The model under review builds one solid part; all positions refer to its coordinate system, in mm. Round coordinates to 2 decimals unless told otherwise and drop trailing zeros. Loops run counter-clockwise (first coordinate to the right, second up) from the corner with the lowest first, then second, coordinate; pieces in that order, holes last. Notation, with made-up numbers: M 24.25,22.25 L 48.25,22.25 A28 cw 48.25,45.25 Z; hole C 66.5,8 d5. An arc over 180 degrees is marked long. Return JSON: item names as keys, results as strings. Group by question number.
Q1. Draft analysis for pull direction Y (two halves, no side actions). For faces 1 (the face through (-103, 406.4, 13)), 2 (the face through (-100.447, 74.932, 16.008)), 3 (the face through (-103, 206, 25.4)), state which applies: pulls with the +Y half, pulls with the -Y half, needs draft (parallel to the pull), parting line crosses it, or undercut.
Q2. Consider section C-C (x = -171.45). State the section outline as (y, z) points.
Q3. To check wall thickness, follow line 1 along X through (y, z) = (387.35, 5) (3 decimals); line 2 along X through (y, z) = (275.5, 15.5); line 3 along Z through (x, y) = (-26.5, 111.5). State the ranges of each line that lie inside material, in increasing order.
Q4. Consider section B-B (y = 261). State the section outline as (x, z) points.
Q5. Clearance check with flat-ended pins moving along their axes: pin 1 Ø10 at (x, y) = (-146, 136) entering from -Z; pin 2 Ø17 at (x, y) = (-114.5, 239) entering from +Z. State where each tip first meets the part, or that it passes through.
Q6. Consider section A-A (z = 14). Count the separate pieces of the cut face and the enclosed holes in it, and give its area (3 significant figures).
Q7. Consider section D-D (y = 217.5). State the section outline as (x, z) points.
from build123d import *

# Parameters (mm, degrees)
F0_W     = 203.2
F0_H     = 406.4
F1_DEPTH = 25.4
F3_DEPTH = 19.05
F4_R     = 3.175
F5_DEPTH = 25.401


with BuildPart() as f1:
    # F0 (on Top) → F1 (new body)
    with BuildSketch(Plane.XY):
        with Locations((-101.6, 203.2)):
            Rectangle(F0_W, F0_H)
    extrude(amount=F1_DEPTH)

    # F2 (on face) → F3 (cut)
    with BuildSketch(Plane.XY.offset(25.4)):
        with BuildLine():
            ThreePointArc((-162.33913, 21.369951), (-101.6, 36.836287), (-40.86087, 21.369951))
            ThreePointArc((-40.86087, 21.369951), (-15.019951, 28.98913), (-22.63913, 54.830049))
            ThreePointArc((-22.63913, 54.830049), (-101.6, 74.936287), (-180.56087, 54.830049))
            ThreePointArc((-180.56087, 54.830049), (-188.180049, 28.98913), (-162.33913, 21.369951))
        make_face()
        with BuildLine():
            ThreePointArc((-162.233016, 84.869862), (-101.493885, 100.336199), (-40.754755, 84.869862))
            ThreePointArc((-40.754755, 84.869862), (-14.913836, 92.489042), (-22.533016, 118.329961))
            ThreePointArc((-22.533016, 118.329961), (-101.493885, 138.436199), (-180.454755, 118.329961))
            ThreePointArc((-180.454755, 118.329961), (-188.073935, 92.489042), (-162.233016, 84.869862))
        make_face()
        with BuildLine():
            ThreePointArc((-162.126901, 148.369773), (-101.387771, 163.83611), (-40.64864, 148.369773))
            ThreePointArc((-40.64864, 148.369773), (-14.807721, 155.988953), (-22.426901, 181.829872))
            ThreePointArc((-22.426901, 181.829872), (-101.387771, 201.93611), (-180.34864, 181.829872))
            ThreePointArc((-180.34864, 181.829872), (-187.96782, 155.988953), (-162.126901, 148.369773))
        make_face()
        with BuildLine():
            ThreePointArc((-162.020787, 211.869685), (-101.281656, 227.336021), (-40.542526, 211.869685))
            ThreePointArc((-40.542526, 211.869685), (-14.701607, 219.488864), (-22.320787, 245.329783))
            ThreePointArc((-22.320787, 245.329783), (-101.281656, 265.436021), (-180.242526, 245.329783))
            ThreePointArc((-180.242526, 245.329783), (-187.861706, 219.488864), (-162.020787, 211.869685))
        make_face()
        with BuildLine():
            ThreePointArc((-161.914672, 275.369596), (-101.175541, 290.835933), (-40.436411, 275.369596))
            ThreePointArc((-40.436411, 275.369596), (-14.595492, 282.988776), (-22.214672, 308.829695))
            ThreePointArc((-22.214672, 308.829695), (-101.175541, 328.935933), (-180.136411, 308.829695))
            ThreePointArc((-180.136411, 308.829695), (-187.755591, 282.988776), (-161.914672, 275.369596))
        make_face()
        with BuildLine():
            ThreePointArc((-161.808557, 338.869507), (-101.069427, 354.335844), (-40.330296, 338.869507))
            ThreePointArc((-40.330296, 338.869507), (-14.489377, 346.488687), (-22.108557, 372.329606))
            ThreePointArc((-22.108557, 372.329606), (-101.069427, 392.435844), (-180.030296, 372.329606))
            ThreePointArc((-180.030296, 372.329606), (-187.649476, 346.488687), (-161.808557, 338.869507))
        make_face()
    extrude(amount=-F3_DEPTH, mode=Mode.SUBTRACT)

    # F4 (on face) → F5 (cut, through all)
    with BuildSketch(Plane.XY.offset(25.4)):
        with Locations((-184.15, 387.35)):
            Circle(F4_R)
        with Locations((-19.05, 387.35)):
            Circle(F4_R)
        with Locations((-184.15, 12.7)):
            Circle(F4_R)
        with Locations((-19.05, 12.7)):
            Circle(F4_R)
    extrude(amount=-F5_DEPTH, mode=Mode.SUBTRACT)


solid = f1.part
Values:
{
 "1": {"face 1": "pulls with the +Y half", "face 2": "undercut", "face 3": "needs draft"},
 "2": {"outline": "M 0,0 L 406.4,0 L 406.4,25.4 L 376.68,25.4 L 376.68,6.35 L 336.56,6.35 L 336.56,25.4 L 313.23,25.4 L 313.23,6.35 L 273.05,6.35 L 273.05,25.4 L 249.78,25.4 L 249.78,6.35 L 209.55,6.35 L 209.55,25.4 L 186.33,25.4 L 186.33,6.35 L 146.05,6.35 L 146.05,25.4 L 122.88,25.4 L 122.88,6.35 L 82.55,6.35 L 82.55,25.4 L 59.43,25.4 L 59.43,6.35 L 19.05,6.35 L 19.05,25.4 L 0,25.4 Z"},
 "3": {"line 1": "x = -203.2 to -187.325, -180.975 to -22.225, -15.875 to 0", "line 2": "x = -203.2 to -180.37, -161.67 to -40.68, -21.98 to 0", "line 3": "z = 0 to 6.35"},
 "4": {"outline": "M -203.2,0 L 0,0 L 0,25.4 L -63.27,25.4 L -63.27,6.35 L -139.3,6.35 L -139.3,25.4 L -203.2,25.4 Z"},
 "5": {"pin 1": "stops at z = 0", "pin 2": "stops at z = 6.35"},
 "6": {"separate pieces": "1", "enclosed holes": "10", "area": "42,300 mm2"},
 "7": {"outline": "M -203.2,0 L 0,0 L 0,25.4 L -15.95,25.4 L -15.95,6.35 L -52.28,6.35 L -52.28,25.4 L -150.29,25.4 L -150.29,6.35 L -186.61,6.35 L -186.61,25.4 L -203.2,25.4 Z"}
}
